Geometry: final body of the model. Coordinates: model frame, mm. Face numbers are marked on the shaded views. A direction names the side the tool comes from. Round coordinates to 2 decimals unless told otherwise and drop trailing zeros. Loops run counter-clockwise (first coordinate to the right, second up) from the corner with the lowest first, then second, coordinate; pieces in that order, holes last. Notation, with made-up numbers: (6, -11) - (36, -11) arc R32 ccw to (36, 27) - close; hole circle Ø11 at (47.25, -29). An arc over 180 degrees is marked (long way). Write item = value, one per line. Start each with the question number.
Item 1: Section B-B (y = 36). Return loops of the section in (x, z).
Item 2: Section C-C (z = 11). Return loops of the section in (x, y).
Item 3: Section D-D (x = 32.5). Return loops of the section in (y, z).
Item 4: First-contact query: pin 1 (1.1 mm diameter, centred on x = 14, y = 21.5, fed in from +Z); pin 2 (0.8 mm diameter, centred on y = 31.5, z = 2, fed in from -X); pin 3 (12 mm diameter, centred on x = -10, y = 14.5, fed in from -Z); pin 4 (2 mm diameter, centred on x = 16, z = 8.5, fed in from -Y). Flat tips, straight axial feed; report the tip coordinate or a pass-through.
Item 5: Line query: line 1 (X direction, y = 33, z = -3); line 2 (Y direction, x = -29, z = -10.5); line 3 (X direction, y = 23, z = -2.5). Output: solid intervals per line, ascending. Write a range as from..to.
Item 6: Access query for the marked faces 5, 6, 7, 8 and 9. Directions: +Z, -Z, +X, -X, +Y, -Y. A direction counts if a zero-diameter tool reaches every point of the face in a straight line with its end or side. Return the directions, or none.
Item 7: Section A-A (y = 29). Return loops of the section in (x, z), plus the area to 3 significant figures.
Item 8: Draft query along X for the marked faces 1, 2, 3 and 4. Return one class per face: pulls with the +X half, pulls with the -X half, needs draft (parallel to the pull), parting line crosses it, or undercut.
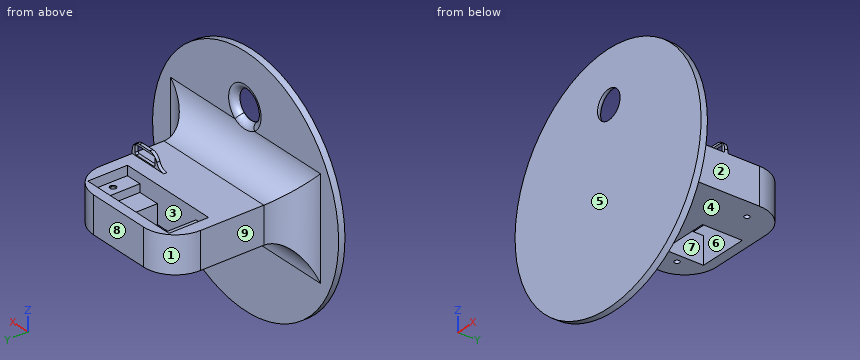
from build123d import *

# Parameters (mm, degrees)
SKETCH1_R                      = 37.25
BOSS_EXTRUDE1_DEPTH            = 2
SKETCH2_W                      = 40
SKETCH2_H                      = 12
BOSS_EXTRUDE4_DEPTH            = 40
SKETCH3_W                      = 32.5
SKETCH3_H                      = 12.5
CUT_EXTRUDE1_DEPTH             = 3
SKETCH4_W                      = 22.5
SKETCH4_H                      = 12.5
CUT_EXTRUDE2_DEPTH             = 2.5
SKETCH5_W                      = 15.5
SKETCH5_H                      = 12.5
CUT_EXTRUDE3_DEPTH             = 6
SKETCH6_W                      = 0.5
SKETCH6_H                      = 40
CUT_EXTRUDE4_DEPTH             = 81.181824624
SKETCH7_R                      = 0.95
CUT_EXTRUDE5_DEPTH             = 0.1
M2X0_4_TAPPED_HOLE1_AT_2_COUNT = 2
M2X0_4_TAPPED_HOLE1_AT_2_PITCH = 28
SKETCH11_W                     = 4
SKETCH11_H                     = 1
BOSS_EXTRUDE9_DEPTH            = 10
CUT_EXTRUDE6_REACH             = 59.089
SKETCH13_W                     = 8
SKETCH13_H                     = 3
FILLET4_R                      = 0.5
FILLET5_R                      = 3
FILLET6_R                      = 3
FILLET7_R                      = 10
FILLET8_R                      = 10
CUT_EXTRUDE7_REACH             = 68.145
SKETCH14_R                     = 4.5
FILLET10_R                     = 2


# Some blends are built 0.0001 mm under size
with BuildPart() as part:
    # Sketch1 → Boss-Extrude1 (new body)
    with BuildSketch(Plane(origin=(0, 0, 0), x_dir=(1, 0, 0), z_dir=(0, 1, 0))):
        with Locations(Location((0, 0, 0), (0, 0, 270))):
            Circle(SKETCH1_R)
    extrude(amount=BOSS_EXTRUDE1_DEPTH)

    # Sketch2 → Boss-Extrude4 (add)
    with BuildSketch(Plane(origin=(0, 2, 0), x_dir=(1, 0, 0), z_dir=(0, 1, 0))):
        Rectangle(SKETCH2_W, SKETCH2_H)
    extrude(amount=BOSS_EXTRUDE4_DEPTH)

    # Sketch3 → Cut-Extrude1 (cut)
    with BuildSketch(Plane.XY.offset(6)):
        with Locations((-0.004059612, 32.710166226)):
            Rectangle(SKETCH3_W, SKETCH3_H)
    extrude(amount=-CUT_EXTRUDE1_DEPTH, mode=Mode.SUBTRACT)

    # Sketch4 → Cut-Extrude2 (cut)
    with BuildSketch(Plane.XY.offset(3)):
        with Locations((-0.004059612, 32.710166226)):
            Rectangle(SKETCH4_W, SKETCH4_H)
    extrude(amount=-CUT_EXTRUDE2_DEPTH, mode=Mode.SUBTRACT)

    # Sketch5 → Cut-Extrude3 (cut)
    with BuildSketch(Plane.XY.offset(0.5)):
        with Locations((-3.504059612, 32.710166226)):
            Rectangle(SKETCH5_W, SKETCH5_H)
    extrude(amount=-CUT_EXTRUDE3_DEPTH, mode=Mode.SUBTRACT)

    # Sketch6 → Cut-Extrude4 (cut, through all)
    with BuildSketch(Plane(origin=(20, 0, 0), x_dir=(0, 0, -1), z_dir=(1, 0, 0))):
        with Locations((5.75, 22)):
            Rectangle(SKETCH6_W, SKETCH6_H)
    extrude(amount=-CUT_EXTRUDE4_DEPTH, mode=Mode.SUBTRACT)

    # Sketch7 → Cut-Extrude5 (cut)
    with BuildSketch(Plane.XY.offset(3)):
        with Locations((14.013948706, 32.755843114)):
            Circle(SKETCH7_R)
        with Locations((-13.986051294, 32.755843114)):
            Circle(SKETCH7_R)
    extrude(amount=-CUT_EXTRUDE5_DEPTH, mode=Mode.SUBTRACT)

    # Sketch9 → M2x0.4 Tapped Hole1 (revolve, cut)
    with BuildSketch(Plane(origin=(-13.986051294, 32.755843114, 2.9), x_dir=(0, -1, 0), z_dir=(1, 0, 0))):
        Polygon((0, 0), (0, 40.15), (0.8, 40.15), (0.8, 0.225), (1.025, 0), align=None)
    m2x0_4_tapped_hole1 = revolve(axis=Axis((-13.986051294, 32.755843114, 9.25), (0, 0, -1)), mode=Mode.SUBTRACT)

    # M2x0.4 Tapped Hole1 at 2: M2x0.4 Tapped Hole1 ×2
    with Locations(*[(i * M2X0_4_TAPPED_HOLE1_AT_2_PITCH, 0, 0) for i in range(1, M2X0_4_TAPPED_HOLE1_AT_2_COUNT)]):
        add(m2x0_4_tapped_hole1, mode=Mode.SUBTRACT)

    # Sketch11 → Boss-Extrude9 (add)
    with BuildSketch(Plane(origin=(20, 0, 0), x_dir=(0, 0, -1), z_dir=(1, 0, 0))):
        with Locations((-8, 21.5)):
            Rectangle(SKETCH11_W, SKETCH11_H)
    extrude(amount=-BOSS_EXTRUDE9_DEPTH)

    # Sketch13 → Cut-Extrude6 (cut, up to next)
    with BuildSketch(Plane(origin=(0, 22, 0), x_dir=(1, 0, 0), z_dir=(0, 1, 0)), mode=Mode.PRIVATE) as cut_extrude6_sk1:
        with Locations((14.894629289, -7.846146156)):
            Rectangle(SKETCH13_W, SKETCH13_H)
    cut_extrude6_tool1 = extrude(cut_extrude6_sk1.sketch, amount=-CUT_EXTRUDE6_REACH, mode=Mode.PRIVATE) & part.part
    add(cut_extrude6_tool1.solids().sort_by_distance((14.894629, 22, 7.846146))[0], mode=Mode.SUBTRACT)

    # Fillet4
    fillet4_edges = [part.edges().sort_by_distance(p)[0] for p in [
        (10.894629289, 21.5, 6.346146156),
        (10.894629289, 21.5, 9.346146156),
        (18.894629289, 21.5, 9.346146156),
        (18.894629289, 21.5, 6.346146156),
    ]]
    fillet(fillet4_edges, radius=FILLET4_R)

    # Fillet5
    fillet5_edges = [part.edges().sort_by_distance(p)[0] for p in [
        (10, 21.5, 10),
        (20, 21.5, 10),
    ]]
    fillet(fillet5_edges, radius=FILLET5_R)

    # Fillet6
    # the kernel refuses this fillet: 3 mm, written as the material it adds along each edge
    with BuildSketch(Plane(origin=(10, 21, 6), x_dir=(0.08547250469841872, 5.30956894242523e-15, 0.9963405296085164), z_dir=(0, 1, 0))) as fillet6_piece_1:
        with BuildLine():
            CenterArc((2.761933602, -2.903549084), FILLET6_R, 104.568024357, 70.528779366)
            Line((-0.227087987, -2.64713157), (-0.525990146, -2.621489819))
            Line((-0.525990146, -2.621489819), (-0.298902159, 0.025641751))
            Line((-0.298902159, 0.025641751), (0.025641751, 0.298902159))
            ThreePointArc((0.025641751, 0.298902159), (1.021982281, 0.213429654), (1.931887045, 0.290354908))
            Line((1.931887045, 0.290354908), (2.007345823, 0))
        make_face()
    extrude(amount=1)

    # Fillet7
    fillet7_edges = [part.edges().sort_by_distance(p)[0] for p in [
        (-20, 2, 0.25),
        (0, 2, -5.5),
        (0, 2, 6),
        (20, 2, 0.25),
    ]]
    fillet(fillet7_edges, radius=FILLET7_R)

    # Fillet8
    fillet8_edges = [part.edges().sort_by_distance(p)[0] for p in [
        (-20, 42, 0.25),
        (20, 42, 0.25),
    ]]
    fillet(fillet8_edges, radius=FILLET8_R)

    # Sketch14 → Cut-Extrude7 (cut, up to next)
    with BuildSketch(Plane(origin=(0, 2, 0), x_dir=(1, 0, 0), z_dir=(0, 1, 0)), mode=Mode.PRIVATE) as cut_extrude7_sk1:
        with Locations(Location((0.293506959, -21.181418859, 0), (0, 0, 270))):
            Circle(SKETCH14_R)
    cut_extrude7_tool1 = extrude(cut_extrude7_sk1.sketch, amount=-CUT_EXTRUDE7_REACH, mode=Mode.PRIVATE) & part.part
    add(cut_extrude7_tool1.solids().sort_by_distance((0.293507, 2, 21.181419))[0], mode=Mode.SUBTRACT)

    # Fillet10
    fillet10_edges = [part.edges().sort_by_distance(p)[0] for p in [
        (0.293506959, 2, 16.681418859),
    ]]
    fillet(fillet10_edges, radius=FILLET10_R - 0.0001)  # a hair under: the kernel refuses the full size


solid = part.part
Taken from the geometry:
q1.outline = (-19.17, -5.5) - (-11.25, -5.5) - (-11.25, 3) - (-16.25, 3) - (-16.25, 6) - (-19.17, 6) - close; (4.25, -5.5) - (19.17, -5.5) - (19.17, 6) - (16.25, 6) - (16.25, 3) - (11.25, 3) - (11.25, 0.5) - (4.25, 0.5) - close
q2.outline = (-35.59, 0) - (35.59, 0) - (35.59, 2) - (30, 2) arc R10 cw to (25, 3.34) - (-25, 3.34) arc R10 cw to (-30, 2) - (-35.59, 2) - close
q3.outline = (0, -18.2) - (2, -18.2) - (2, 18.2) - (0, 18.2) - close
q4.pin_1 = 10
q4.pin_2 = -20
q4.pin_3 = -6.13
q4.pin_4 = 0
q5.line_1 = -19.95..-14.75, -13.22..-11.25, 4.25..13.25, 14.78..19.95
q5.line_2 = 0..2.05
q5.line_3 = -20..20
q6.face_5 = +Z, -Z, +X, -X, -Y
q6.face_6 = +Z
q6.face_7 = +Z, -Z
q6.face_8 = +Z, -Z, +X, -X, +Y
q6.face_9 = +Z, -Z, -X, +Y
q7.outline = (-20, -5.5) - (-11.25, -5.5) - (-11.25, 3) - (-16.25, 3) - (-16.25, 6) - (-20, 6) - close; (4.25, -5.5) - (20, -5.5) - (20, 6) - (16.25, 6) - (16.25, 3) - (11.25, 3) - (11.25, 0.5) - (4.25, 0.5) - close
q7.area = 213 mm^2
q8.face_1 = pulls with the -X half
q8.face_2 = pulls with the +X half
q8.face_3 = undercut
q8.face_4 = needs draft
